Part model, mm, in its own coordinate system. A direction names the side the tool comes from. Coordinates: 2 decimals unless noted, no trailing zeros. Order: outer loops, then holes, each group sorted by start corner. A loop starts at its lowest first (then second) coordinate and runs counter-clockwise, first axis right, second up.
Autodesk Inventor part; units mm, degrees
ref_plane "YZ Plane" through (0, 0, 0) normal (1, 0, 0) x (0, 1, 0)
ref_plane "XZ Plane" through (0, 0, 0) normal (0, 1, 0) x (-1, 0, 0)
ref_plane "XY Plane" through (0, 0, 0) normal (0, 0, 1) x (1, 0, 0)
sketch "Sketch1" plane through (0, 0, 0) normal (0, 0, 1) x (1, 0, 0)
  line L0 (42.72, 0) -> (42.72, 77.18)
  line L1 (42.72, 77.18) -> (0, 77.18)
  line L2 (0, 77.18) -> (0, 0)
  line L3 (0, 0) -> (42.72, 0)
  point P0 (0, 0)
  dimension "d0" = 77.18
  dimension "d1" = 42.72
extrude "Extrusion1" add sketch "Sketch1" along normal blind 2
sketch "Sketch3" plane through (0, 0, 2) normal (0, 0, 1) x (1, 0, 0)
  line L0 (1.3486, 0.5) -> (41.3486, 0.5)
  line L1 (41.3486, 0.5) -> (41.3486, 3.5)
  line L2 (41.3486, 3.5) -> (1.3486, 3.5)
  line L3 (1.3486, 3.5) -> (1.3486, 0.5)
  line L4 (0, 0) -> (42.72, 0)
  dimension "d4" = 40
  dimension "d5" = 3
  dimension "d18" = 0.5
sketch "Sketch4" plane through (0, 0, 2) normal (0, 0, 1) x (1, 0, 0)
  point P0 (0, 0)
sketch "Sketch5" plane through (0, 0, 2) normal (0, 0, 1) x (1, 0, 0)
  point P0 (0, 0)
extrude "Extrusion2" add sketch "Sketch3" along normal blind 2.54
sketch "Sketch6" plane through (-2.2901, 18.5965, 2) normal (0, 0, 1) x (1, 0, 0)
  line L0 (41.636, -17.8665) -> (41.636, -16.2696)
  line L1 (41.636, -16.2696) -> (6, -16.2696)
  line L2 (6, -16.2696) -> (6, -17.8665)
  line L3 (6, -17.8665) -> (41.636, -17.8665)
  line L4 (43.6387, -18.0965) -> (3.6387, -18.0965)
  point P0 (0, 0)
  dimension "d19" = 0.23
extrude "Extrusion3" add sketch "Sketch6" along normal blind 10.54
sketch "Sketch7" plane through (0, 0, 2) normal (0, 0, 1) x (1, 0, 0)
  circle A0 centre (3, 6.92) radius 1.6
  point P0 (0, 0)
  dimension "d11" = 3.2
extrude "Extrusion4" cut sketch "Sketch7" against normal blind 2.54
sketch "Sketch8" plane through (0, 0, 2) normal (0, 0, 1) x (1, 0, 0)
  circle A0 centre (3, 74.18) radius 1.6
  circle A1 centre (39.72, 74.18) radius 1.6
  point P0 (0, 0)
  dimension "d14" = 3.2
extrude "Extrusion5" cut sketch "Sketch8" against normal blind 2.54
properties part number "lcd display"
Q1. Wall check: line 1 along X through (y, z) = (74.18, 0.85); line 2 along Y through (x, z) = (3, 0.6); line 3 along Y through (x, z) = (39.72, 0.6). Give the ranges that are in metal, low to high.
Results list:
line 1: x = 0 to 1.4, 4.6 to 38.12, 41.32 to 42.72
line 2: y = 0 to 5.32, 8.52 to 72.58, 75.78 to 77.18
line 3: y = 0 to 72.58, 75.78 to 77.18
Q2. Cut at B-B on y = 6.92. Write the cut outline in (x, z), and give its area (3 significant figures).
Results list:
outline: (0, 0) - (1.4, 0) - (1.4, 2) - (0, 2) - close; (4.6, 0) - (42.72, 0) - (42.72, 2) - (4.6, 2) - close
area: 79.0 mm2
Q3. Cut at C-C on x = 33. Write the cut outline in (y, z).
Results list:
outline: (0, 0) - (77.18, 0) - (77.18, 2) - (3.5, 2) - (3.5, 4.54) - (2.33, 4.54) - (2.33, 12.54) - (0.73, 12.54) - (0.73, 4.54) - (0.5, 4.54) - (0.5, 2) - (0, 2) - close
Q4. Which spindle directions (+Z, -Z, +X, -X, +Y, -Y) get a long thin tool onto all of the face, cutting with end or side? Do faces 4 (the face through (1.349, 2, 3)), 5 (the face through (39.346, 2, 8)), 6 (the face through (22, 3.5, 3)), 7 (the face through (2.65, 72.62, 1.01)), 8 (the face through (21, 0.5, 3)). Say none if no direction does.
Results list:
face 4: +Z, -X, +Y, -Y
face 5: +Z, +X, +Y, -Y
face 6: +Z, +X, -X, +Y
face 7: +Z, -Z
face 8: +Z, +X, -X, -Y
Q5. Cut at D-D on z = 7.75. Write the cut outline in (x, y), and give its area (3 significant figures).
Results list:
outline: (3.71, 0.73) - (39.35, 0.73) - (39.35, 2.33) - (3.71, 2.33) - close
area: 56.9 mm2
Q6. Cut at A-A on y = 74.18. Write the cut outline in (x, z), and give its area (3 significant figures).
Results list:
outline: (0, 0) - (1.4, 0) - (1.4, 2) - (0, 2) - close; (4.6, 0) - (38.12, 0) - (38.12, 2) - (4.6, 2) - close; (41.32, 0) - (42.72, 0) - (42.72, 2) - (41.32, 2) - close
area: 72.6 mm2
Q7. Mould opens along Y. For faces 1 (the face through (21, 0.73, 8)), 2 (the face through (21, 39, 0)), 3 (the face through (39.37, 72.62, 1.01)) say: pulls with the +Y half, pulls with the -Y half, needs draft (parallel to the pull), parting line crosses it, or undercut.
Results list:
face 1: pulls with the -Y half
face 2: needs draft
face 3: undercut
Q8. Pin check, flat tips, straight feed: pin 1 Ø0.5 at (y, z) = (1.5, 7.5) entering from +X; pin 2 Ø5 at (x, y) = (33.5, 35.5) entering from +Z; pin 3 Ø0.5 at (y, z) = (2, 8) entering from -X. Stop position of each tip, or through.
Results list:
pin 1: stops at x = 39.35
pin 2: stops at z = 2
pin 3: stops at x = 3.71
